Here's how the part is built. I have some questions about the finished solid (model axes, mm). Face numbers are marked on the shaded views. A direction names the side the tool comes from. Coordinates: 2 decimals unless noted, no trailing zeros. Loops run counter-clockwise (first coordinate to the right, second up) from the corner with the lowest first, then second, coordinate; pieces in that order, holes last. Notation, with made-up numbers: (4, -23.5) -> (36, -23.5) arc R12 cw to (36, -17.5) -> close; hole circle Ø5 at (25.5, -27). An arc over 180 degrees is marked (long way). Answer as a JSON object with one key per item and string values. Group by question number.
1) I need wall thicknesses on probe 1 along X at (y, z) = (3.5, 0); probe 2 along X at (y, z) = (9.25, -2); probe 3 along Z at (x, y) = (0.75, 11.25). Which ranges of each line are inside material? Lowest first, please. Write a range as [from, to].
2) I want a section at D-D (y = 1.25). Write out the boundary of the cut face in (x, z) (3 decimals), then the cut area to 3 significant figures.
3) Which directions (+Z, -Z, +X, -X, +Y, -Y) give clear straight access to the entire face, cutting with the end or side of a thin tool? Please do the marked faces 4 and 5.
4) I want a section at C-C (y = 3). Write out the boundary of the cut face in (x, z), then the cut area to 3 significant figures.
5) I'm going to push flat-ended pins straight in: pin 1 (6 mm diameter, centred on x = 0, z = -1, fed in from +Y); pin 2 (2 mm diameter, centred on x = -1, z = 1, fed in from -Y); pin 3 (2 mm diameter, centred on x = -1.5, y = 2.5, fed in from -Z); pin 4 (3 mm diameter, centred on y = 11, z = 3.5, fed in from -X). Where does each tip first touch, or does it pass through?
6) If we mould it in two halves opening along Z, with no side actions, what happens to the marked faces 1, 2 and 3? For each: +Z half, -Z half, draft (parallel to the pull), parting line (faces both ways), or undercut.
7) I want a section at B-B (x = 0). Write out the boundary of the cut face in (y, z), then the cut area to 3 significant figures.
8) I want a section at A-A (z = 0). Write out the boundary of the cut face in (x, y), then the cut area to 3 significant figures.
```python
from build123d import *

# Parameters (mm, degrees)
SKETCH_1_R       = 5
SKETCH_1_R_2     = 3
EXTRUDE_1_DEPTH  = 13
SKETCH_1_3_R     = 6
SKETCH_1_3_R_2   = 5
EXTRUDE_2_DEPTH  = 2
CHAMFER_1_SIZE   = 1
CHAMFER_1_SIZE_2 = 2


with BuildPart() as part:
    # 草图1 → 凸台-拉伸1 (new body)
    with BuildSketch(Plane(origin=(0, 0, 0), x_dir=(1, 0, 0), z_dir=(0, 1, 0))):
        with Locations(Location((0, 0, 0), (0, 0, 90))):
            Circle(SKETCH_1_R)
        with Locations(Location((0, 0, 0), (0, 0, 90))):
            Circle(SKETCH_1_R_2, mode=Mode.SUBTRACT)
    extrude(amount=EXTRUDE_1_DEPTH)

    # 草图1<3> → 凸台-拉伸2 (add)
    with BuildSketch(Plane(origin=(0, 0, 0), x_dir=(1, 0, 0), z_dir=(0, 1, 0))):
        with Locations(Location((0, 0, 0), (0, 0, 270))):
            Circle(SKETCH_1_3_R)
        with Locations(Location((0, 0, 0), (0, 0, 90))):
            Circle(SKETCH_1_3_R_2, mode=Mode.SUBTRACT)
    extrude(amount=EXTRUDE_2_DEPTH)

    # 倒角1
    # the kernel refuses this chamfer: 2, 1 mm, written as the material it takes off along each edge
    with BuildSketch(Plane(origin=(0, 2, 0), x_dir=(0, 0, 1), z_dir=(-1, 0, 0))) as chamfer_1_piece_1:
        Polygon((6 - CHAMFER_1_SIZE, 0), (6, -CHAMFER_1_SIZE_2), (6, 0), align=None)
    revolve(axis=Axis((0, 2, 0), (0, 1, 0)), mode=Mode.SUBTRACT)


solid = part.part
```
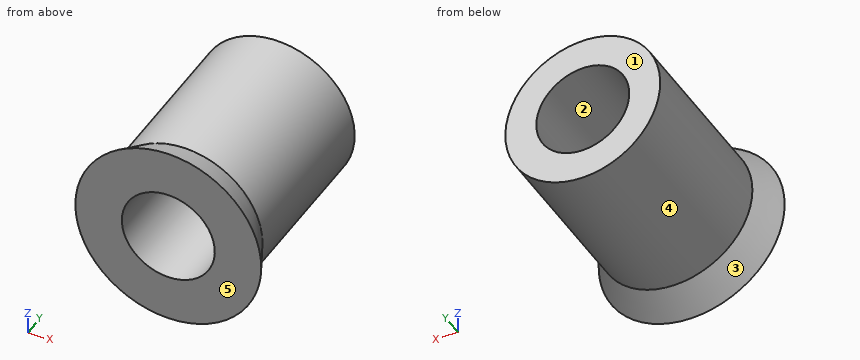
Determined:
{
 "1": {"probe 1": "[-5, -3], [3, 5]", "probe 2": "[-4.58, -2.24], [2.24, 4.58]", "probe 3": "[-4.94, -2.9], [2.9, 4.94]"},
 "2": {"outline": "circle Ø10.75 at (0, 0); hole circle Ø6 at (0, 0)", "area": "62.5 mm^2"},
 "3": {"face 4": "+Y", "face 5": "+Z, -Z, +X, -X, -Y"},
 "4": {"outline": "circle Ø10 at (0, 0); hole circle Ø6 at (0, 0)", "area": "50.3 mm^2"},
 "5": {"pin 1": "y = 13", "pin 2": "through", "pin 3": "z = -5.09", "pin 4": "x = -4.58"},
 "6": {"face 1": "draft", "face 2": "undercut", "face 3": "parting line"},
 "7": {"outline": "(0, -6) -> (2, -5) -> (13, -5) -> (13, -3) -> (0, -3) -> close; (0, 3) -> (13, 3) -> (13, 5) -> (2, 5) -> (0, 6) -> close", "area": "54.0 mm^2"},
 "8": {"outline": "(-6, 0) -> (-3, 0) -> (-3, 13) -> (-5, 13) -> (-5, 2) -> close; (3, 0) -> (6, 0) -> (5, 2) -> (5, 13) -> (3, 13) -> close", "area": "54.0 mm^2"}
}
